Read the model definition and answer for the solid it produces. Units are mm, in the model's axes. Face numbers are marked on the shaded views. A direction names the side the tool comes from. Coordinates: 2 decimals unless noted, no trailing zeros. Order: outer loops, then holes, each group sorted by start corner. A loop starts at its lowest first (then second) coordinate and runs counter-clockwise, first axis right, second up. Notation, with made-up numbers: (79, 70) -> (117, 70) arc R27 cw to (117, 109) -> close; hole circle Ø10 at (59.25, -11.75). An arc over 180 degrees is marked (long way). Answer as a JSON object with one key per item and string values. Group by question number.
1) A tool of negligible diameter and unlimited length cuts with its end or side. For the marked faces 1 and 2, from which of +Z, -Z, +X, -X, +Y, -Y can it reach the whole face along a straight path? Write none if from no direction.
2) Section B-B on y = 10 is taken. Determine the outline of the cut face in (x, z), and give its area (3 significant figures).
3) Section C-C on z = 10 is taken. Determine the outline of the cut face in (x, y), and give its area (3 significant figures).
4) Given pin 1 (2.5 mm diameter, centred on y = 6.5, z = 6.5, fed in from -X); pin 2 (6.5 mm diameter, centred on x = -12.5, y = 7.5, fed in from +Z); pin 3 (6.5 mm diameter, centred on x = -47.5, y = 6, fed in from +Z), each flat-ended and moving along its own axis, determine where each tip first touches the part or whether it passes through.
5) Determine the mould class of the marked faces 3 and 4 for opening direction X: released by +X, released by -X, zero draft, split by the parting line, or undercut.
6) Consider L1, parallel to Z at x = -8.5, y = 6.25; L2, parallel to Y at x = -30.5, z = 3.25; L3, parallel to Y at x = -39, z = 10. Determine where each line is inside the solid, lowest interval first.
7) Section A-A on y = 7 is taken. Determine the outline of the cut face in (x, z), and give its area (3 significant figures).
8) Section D-D on x = -46 is taken. Determine the outline of the cut face in (y, z).
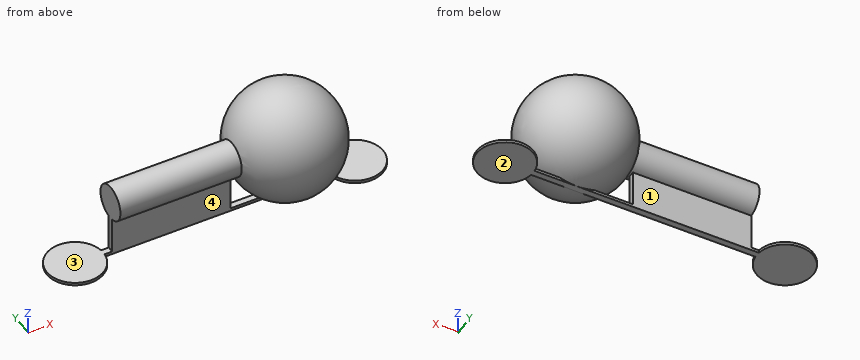
from build123d import *

# Parameters (mm, degrees)
EXTRUDE_DEPTH  = 0.4
CYLINDER_R     = 2.5
CYLINDER_DEPTH = 25
BOX_W          = 17
BOX_H          = 0.9
BOX_DEPTH      = 8


with BuildPart() as extrude_body:
    # Sketch011 (on Face6 of Fusion) → Extrude (new body)
    with BuildSketch(Plane(origin=(0, 0, 2), x_dir=(1, 0, 0), z_dir=(0, 0, -1))):
        with BuildLine():
            Line((-44.094311, -6.55), (-11.902384, -6.55))
            ThreePointArc((-11.902384, -7.45), (-3.927777, -7), (-11.902384, -6.55))
            Line((-11.902384, -7.45), (-44.094311, -7.45))
            ThreePointArc((-44.094311, -6.55), (-52.068918, -7), (-44.094311, -7.45))
        make_face()
    extrude(amount=-EXTRUDE_DEPTH)


with BuildPart() as cylinder:
    # Cylinder → Cylinder (new body)
    with BuildSketch(Plane(origin=(-18, 7, 10), x_dir=(0, 0, 1), z_dir=(-1, 0, 0))):
        Circle(CYLINDER_R)
    extrude(amount=CYLINDER_DEPTH)


with BuildPart() as cube:
    # Box → Box (new body)
    with BuildSketch(Plane(origin=(-43, 6.55, 2), x_dir=(1, 0, 0), z_dir=(0, 0, 1))):
        with Locations((8.5, 0.45)):
            Rectangle(BOX_W, BOX_H)
    extrude(amount=BOX_DEPTH)


with BuildPart() as ball:
    # Sphere001 → Sphere001 (revolve)
    with BuildSketch(Plane(origin=(-18, 7, 10), x_dir=(1, 0, 0), z_dir=(0, -1, 0))):
        with BuildLine():
            ThreePointArc((0, -8), (8, 0), (0, 8))
            Line((0, 8), (0, -8))
        make_face()
    revolve(axis=Axis((-18, 7, 10), (0, 0, 1)))

    # Fusion: union Cylinder, Cube
    add(cylinder.part)
    add(cube.part)

    # Fusion001: union Extrude body
    add(extrude_body.part)


solid = ball.part
Worked answers:
{
 "1": {"face 1": "-Z, +Y", "face 2": "-Z, +X, -X, +Y, -Y"},
 "2": {"outline": "(-50.71, 2) -> (-45.42, 2) -> (-45.42, 2.4) -> (-50.71, 2.4) -> close; circle Ø14.83 at (-18, 10); (-10.57, 2) -> (-5.28, 2) -> (-5.28, 2.4) -> (-10.57, 2.4) -> close", "area": "177 mm²"},
 "3": {"outline": "(-43, 4.5) -> (-25.6, 4.5) arc R8 ccw (long way) to (-25.6, 9.5) -> (-43, 9.5) -> close", "area": "287 mm²"},
 "4": {"pin 1": "stops at x = -43", "pin 2": "stops at z = 17.67", "pin 3": "stops at z = 2.4"},
 "5": {"face 3": "zero draft", "face 4": "undercut"},
 "6": {"L1": "z = 2 to 2.4", "L2": "y = 6.55 to 7.45", "L3": "y = 4.5 to 9.5"},
 "7": {"outline": "(-52.07, 2) -> (-3.93, 2) -> (-3.93, 2.4) -> (-15.5, 2.4) arc R8 ccw (long way) to (-25.6, 12.5) -> (-43, 12.5) -> (-43, 2.4) -> (-52.07, 2.4) -> close; hole (-26, 2.4) -> (-20.5, 2.4) arc R8 cw to (-25.6, 7.5) -> (-26, 7.5) -> close", "area": "391 mm²"},
 "8": {"outline": "(3.58, 2) -> (10.42, 2) -> (10.42, 2.4) -> (3.58, 2.4) -> close"}
}
